from build123d import *

# Parameters (mm, degrees)
F3_DEPTH = 12.7


with BuildPart() as f1:
    # F0 (on Front) → F1 (revolve)
    with BuildSketch(Plane.XZ):
        with BuildLine():
            Line((0, 30.48), (0, 2.921))
            Line((0, 2.921), (4.02617, 2.921))
            Line((4.02617, 2.921), (5.29617, 4.191))
            Line((5.29617, 4.191), (5.29617, 18.034))
            Line((5.29617, 18.034), (17.99617, 18.034))
            Line((17.99617, 18.034), (17.99617, 23.368))
            ThreePointArc((17.99617, 23.368), (11.049548, 25.266883), (6.034837, 30.435439))
            ThreePointArc((6.034837, 30.435439), (5.102088, 31.396803), (3.81, 31.75))
            Line((3.81, 31.75), (1.27, 31.75))
            ThreePointArc((1.27, 31.75), (0.371974, 31.378026), (0, 30.48))
        make_face()
    revolve(axis=Axis((18.239362, 0, 0), (1, 0, 0)))

    # F2 (on face) → F3 (cut, through all)
    with BuildSketch(Plane.YZ.offset(17.99617)):
        with BuildLine():
            Line((-18.034, 36.491495), (-18.034, 0))
            ThreePointArc((-18.034, 0), (0, -18.034), (18.034, 0))
            Line((18.034, 0), (18.034, 36.491495))
            Line((18.034, 36.491495), (-18.034, 36.491495))
        make_face()
    extrude(amount=-F3_DEPTH, mode=Mode.SUBTRACT)


solid = f1.part
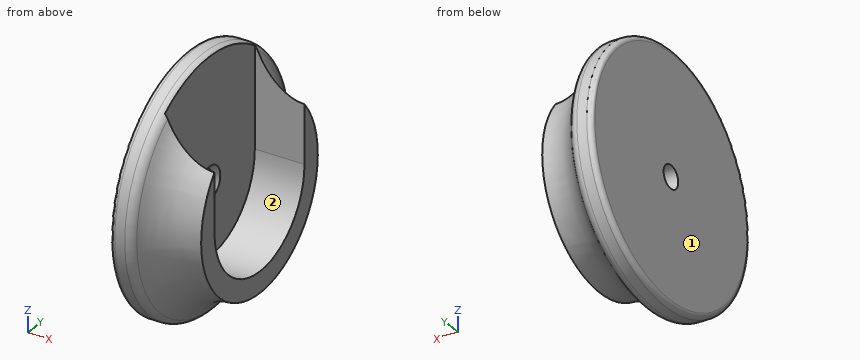
Verification items for the finished model (mm, model axes). Face numbers are marked on the shaded views. A direction names the side the tool comes from. Give positions to 0.01 mm unless a question says otherwise; leave off trailing zeros. Loops run counter-clockwise (first coordinate to the right, second up) from the corner with the lowest first, then second, coordinate; pieces in that order, holes last.
1) Sectioned sample at A-A, the plane y = 0. Enter the section's corners in (x, z).
2) Depth check by flat-ended pin: pin 1 Ø1 at (y, z) = (-6, 7.5) entering from +X; pin 2 Ø4 at (x, z) = (8.5, -8.5) entering from +Y; pin 3 Ø7.5 at (y, z) = (0, 0) entering from +X; pin 4 Ø8 at (y, z) = (14, 7.5) entering from -X. Enter the tip coordinate at first touch or a pass-through.
3) Sectioned sample at B-B, the plane x = 13.25. Enter the section's corners in (y, z), then the cut area to 3 significant figures.
4) Set-up check for the marked faces 1 and 2: record each of +Z, -Z, +X, -X, +Y, -Y from which the full face is reachable in a straight line by a thin tool's end or side.
5) Thickness scan on line 1 along Y through (x, z) = (1.25, 0); line 2 along X through (y, z) = (-14, 4). Record the ranges inside material, lowest first.
Answers:
1. outline: (0, -30.48) arc R1.27 ccw to (1.27, -31.75) - (3.81, -31.75) arc R2.54 ccw to (6.03, -30.44) arc R13.66 cw to (18, -23.37) - (18, -18.03) - (5.3, -18.03) - (5.3, -4.19) - (4.03, -2.92) - (0, -2.92) - close; (0, 2.92) - (4.03, 2.92) - (5.3, 4.19) - (5.3, 31.27) arc R2.54 ccw to (3.81, 31.75) - (1.27, 31.75) arc R1.27 ccw to (0, 30.48) - close
2. pin 1: stops at x = 5.3
2. pin 2: stops at y = 28.46
2. pin 3: stops at x = 4.86
2. pin 4: stops at x = 0
3. outline: (-18.03, 0) - (-18.03, 16.17) arc R24.22 ccw (long way) to (18.03, 16.17) - (18.03, 0) arc R18.03 cw to start
3. area: 548 mm2
4. face 1: +Z, -Z, -X, +Y, -Y
4. face 2: +Z, +X
5. line 1: y = -31.75 to -2.92, 2.92 to 31.75
5. line 2: x = 0 to 5.3
